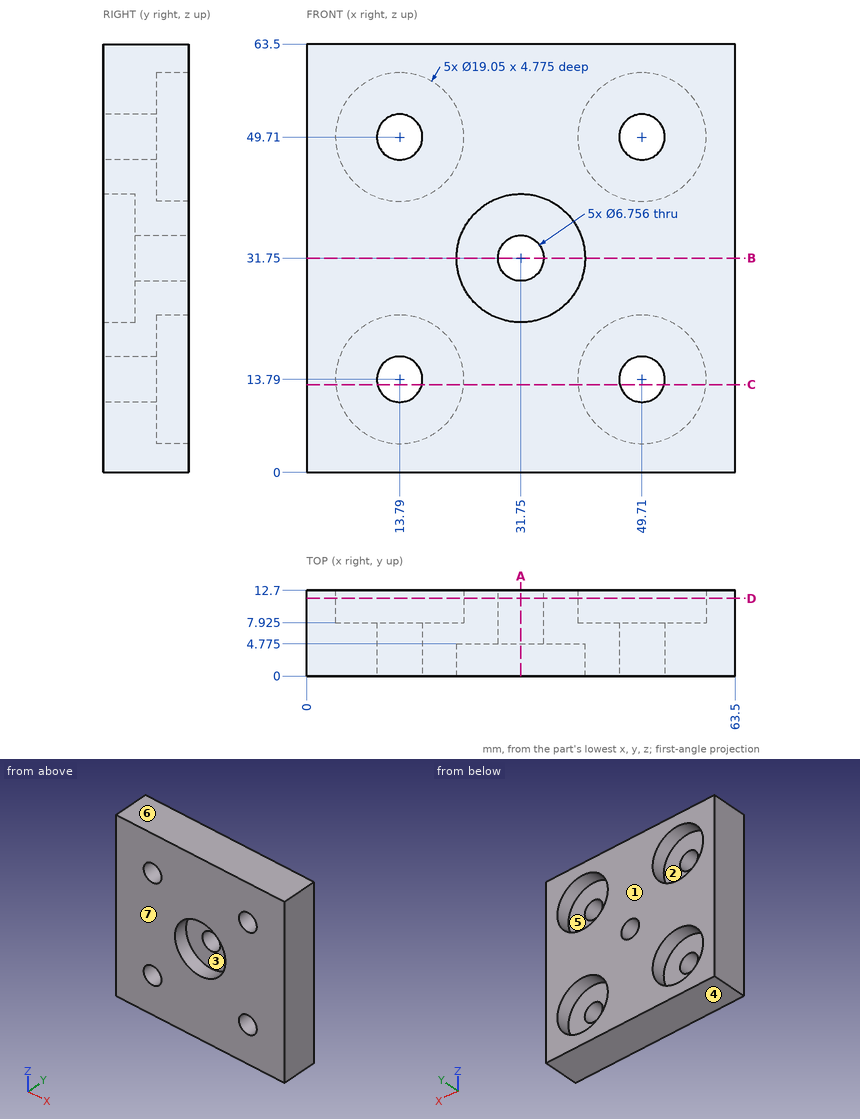
Check sheet for the drawn part. Datum: minimum x, y, z corner. Units: mm. A direction names the side the tool comes from. Give positions to 0.01 mm unless a question says otherwise; leave off trailing zeros. Loops run counter-clockwise (first coordinate to the right, second up) from the corner with the lowest first, then second, coordinate; pieces in that order, holes last.
1) Sectioned sample at A-A, the plane x = 31.75. Enter the section's corners in (y, z) (1 decimal), then the cut area to 3 significant figures.
2) Sectioned sample at D-D, the plane y = 11.5. Count the separate pieces of the cut face and the enclosed holes in it, then the cut area to 3 significant figures.
3) Set-up check for the marked faces 1, 2 and 3: record each of +Z, -Z, +X, -X, +Y, -Y from which the full face is reachable in a straight line by a thin tool's end or side.
4) Sectioned sample at C-C, the plane z = 13. Enter the section's corners in (x, y) (1 decimal), then the cut area to 3 significant figures.
5) Thickness scan on line 1 along Z through (x, y) = (31.75, 10.5); line 2 along X through (y, z) = (4, 32); line 3 along Z through (x, y) = (31.75, 3.2) (1 decimal). Record the ranges inside material, lowest first.
6) Depth check by flat-ended pin: pin 1 Ø1.5 at (x, y) = (57, 10) entering from -Z; pin 2 Ø6 at (x, z) = (46, 17) entering from +Y (1 decimal); pin 3 Ø15 at (x, z) = (31.75, 31.75) entering from -Y (1 decimal). Enter the tip coordinate at first touch or a pass-through.
7) Draft check along Z on the marked faces 4, 5, 6 and 7. Enter one of: pulls with the +Z half, pulls with the -Z half, needs draft (parallel to the pull), parting line crosses it, or undercut.
8) Sectioned sample at B-B, the plane z = 31.75. Enter the section's corners in (x, y) (1 decimal), then the cut area to 3 significant figures.
Answers:
1. outline: (0, 0) - (12.7, 0) - (12.7, 28.4) - (4.8, 28.4) - (4.8, 22.2) - (0, 22.2) - close; (0, 41.3) - (4.8, 41.3) - (4.8, 35.1) - (12.7, 35.1) - (12.7, 63.5) - (0, 63.5) - close
1. area: 662 mm2
2. separate pieces: 1
2. enclosed holes: 5
2. area: 2,860 mm2
3. face 1: +Z, -Z, +X, -X, +Y
3. face 2: +Y
3. face 3: -Y
4. outline: (0, 0) - (10.5, 0) - (10.5, 7.9) - (4.3, 7.9) - (4.3, 12.7) - (0, 12.7) - close; (17.1, 0) - (46.4, 0) - (46.4, 7.9) - (40.2, 7.9) - (40.2, 12.7) - (23.3, 12.7) - (23.3, 7.9) - (17.1, 7.9) - close; (53, 0) - (63.5, 0) - (63.5, 12.7) - (59.2, 12.7) - (59.2, 7.9) - (53, 7.9) - close
4. area: 521 mm2
5. line 1: z = 0 to 28.37, 35.13 to 63.5
5. line 2: x = 0 to 22.23, 41.27 to 63.5
5. line 3: z = 0 to 22.2, 41.3 to 63.5
6. pin 1: stops at z = 0
6. pin 2: stops at y = 7.9
6. pin 3: stops at y = 4.8
7. face 4: pulls with the -Z half
7. face 5: undercut
7. face 6: pulls with the +Z half
7. face 7: needs draft
8. outline: (0, 0) - (22.2, 0) - (22.2, 4.8) - (28.4, 4.8) - (28.4, 12.7) - (0, 12.7) - close; (35.1, 4.8) - (41.3, 4.8) - (41.3, 0) - (63.5, 0) - (63.5, 12.7) - (35.1, 12.7) - close
8. area: 662 mm2
